Autodesk Inventor part; units mm, degrees
ref_plane "YZ Plane" through (0, 0, 0) normal (1, 0, 0) x (0, 1, 0)
ref_plane "XZ Plane" through (0, 0, 0) normal (0, 1, 0) x (-1, 0, 0)
ref_plane "XY Plane" through (0, 0, 0) normal (0, 0, 1) x (1, 0, 0)
sketch "Skizze1" plane through (0, 0, 0) normal (0, 1, 0) x (-1, 0, 0)
  line L0 (0, -10) -> (0, 10)
  line L1 (0, 10) -> (40, 10)
  line L2 (40, 10) -> (50, 0)
  line L3 (50, 0) -> (50, -7)
  line L4 (50, -7) -> (35, -7)
  line L5 (35, -7) -> (35, -10)
  line L6 (35, -10) -> (0, -10)
  line L7 (0, 0) -> (85.3703, 0) construction
  dimension "d0" = 10
  dimension "d1" = 10
  dimension "d2" = 3
  dimension "d3" = 20
  dimension "d4" = 40
  dimension "d5" = 15
extrude "Extrusion1" add sketch "Skizze1" along normal blind 60
sketch "Skizze2" plane through (-35, 0, -7) normal (0, 0, -1) x (-1, 0, 0)
  line L0 (15, 0) -> (15, 60)
  line L1 (15, 30) -> (5.3736, 30) construction
  line L2 (0, 60) -> (15, 60)
  point P0 (-35, 0)
  point P1 (8, 10)
  point P2 (8, 50)
  dimension "d8" = 7
  dimension "d9" = 7
  dimension "d10" = 40
  dimension "d11" = 10
hole "Bohrung1" at (-43, 10, -7) at (-43, 50, -7) direction (0, 0, 1) diameter 3.242 depth 12 tip angle 118
sketch "Skizze3" plane through (0, 0, -10) normal (0, 0, -1) x (-1, 0, 0)
  line L0 (0, 0) -> (0, 60)
  line L1 (0, 0) -> (35, 0)
  point P0 (20, 52)
  point P1 (20, 30)
  point P2 (20, 12)
  point P3 (0, 30)
  dimension "d19" = 20
  dimension "d20" = 12
  dimension "d21" = 40
hole "Bohrung2" at (-20, 12, -10) at (-20, 52, -10) direction (0, 0, 1) diameter 14 depth 20
hole "Bohrung3" at (-20, 30, -10) direction (0, 0, 1) diameter 13.835 depth 20
sketch "Skizze6" plane through (0, 0, 10) normal (1, 0, 0) x (0, 0, -1)
  line L0 (0, 60) -> (20, 60)
  point P0 (10, 0)
  point P1 (10, 54.0188)
  point P2 (10, 60)
hole "Bohrung4" at (0, 54.0188, 0) direction (-1, 0, 0) diameter 4.134 depth 10 tip angle 118
sketch "Skizze7" plane through (0, 0, 10) normal (1, 0, 0) x (0, 0, -1)
  line L0 (0, 0) -> (20, 0)
  point P0 (10, 0)
  point P1 (10, 10)
  point P2 (10, 0)
  point P3 (10, 0)
  dimension "d51" = 10
hole "Bohrung5" at (0, 10, 0) direction (-1, 0, 0) diameter 4.134 depth 10 tip angle 118
sketch "Skizze8" plane through (0, 0, 10) normal (1, 0, 0) x (0, 0, -1)
  line L0 (0, 0) -> (20, 0)
  point P0 (10, 0)
  point P1 (10, 30)
  point P2 (10, 0)
  point P3 (10, 0)
  point P4 (10, 0)
  dimension "d59" = 30
hole "Bohrung6" at (0, 30, 0) direction (-1, 0, 0) diameter 4.134 depth 10 tip angle 118
properties part number "spannbakce"
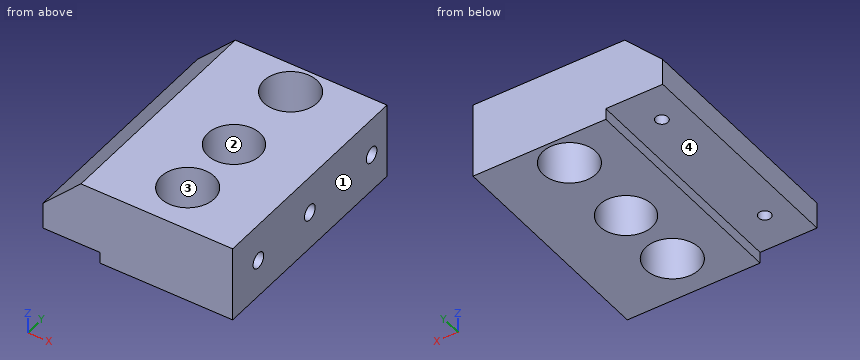
Can you work these out from the model? Positions are in its coordinate system, mm. Face numbers are marked on the shaded views. Coordinates: 2 decimals unless noted, no trailing zeros. Order: outer loops, then holes, each group sorted by start corner. A loop starts at its lowest first (then second) coordinate and runs counter-clockwise, first axis right, second up. Notation, with made-up numbers: (-4, -5.5) -> (0, -5.5) arc R17 cw to (0, 15.5) -> close; hole circle Ø3 at (-38.5, 48). An arc over 180 degrees is marked (long way). Use one line per item in the form item = value.
Q1. Will these pins go through, and if not, where does the flat tip stop? P1, Ø12.5, axis at x = -20, y = 30, coming from the -Z side; P2, Ø2, axis at x = -41.5, y = 30.5, coming from the -Z side; P3, Ø3, axis at y = 23, z = 4.5, coming from the -X side; P4, Ø3, axis at x = -43, y = 50, coming from the -Z side.
From the geometry:
P1 = through
P2 = -7
P3 = -47
P4 = 5.07
Q2. I need wall thicknesses on L1, parallel to Y at x = -20, z = -1.25; L2, parallel to Y at x = -2.75, z = 0; L3, parallel to Z at x = -5, y = 30. Which ranges of each line are inside material? Lowest first, please.
From the geometry:
L1 = 0 to 5, 19 to 23.08, 36.92 to 45, 59 to 60
L2 = 0 to 7.93, 12.07 to 27.93, 32.07 to 51.95, 56.09 to 60
L3 = -10 to -2.07, 2.07 to 10
Q3. Imagine slicing it at D-D, the plane z = 7.75. Give the number of separate pieces and of enclosed holes in the cut face, then the cut area to 3 significant figures.
From the geometry:
separate_pieces = 1
enclosed_holes = 3
area = 2,080 mm²
Q4. Imagine slicing it at A-A, the plane z = -5.5. List the corners of the cut face in (x, y) for me (1 decimal), then the cut area to 3 significant figures.
From the geometry:
outline = (-50, 0) -> (0, 0) -> (0, 60) -> (-50, 60) -> close; hole circle Ø3.2 at (-43, 10); hole circle Ø3.2 at (-43, 50); hole circle Ø14 at (-20, 12); hole circle Ø14 at (-20, 52); hole circle Ø13.8 at (-20, 30)
area = 2,530 mm²
Q5. Imagine slicing it at B-B, the plane x = -20. List the corners of the cut face in (y, z) for me, then the cut area to 3 significant figures.
From the geometry:
outline = (0, -10) -> (5, -10) -> (5, 10) -> (0, 10) -> close; (19, -10) -> (23.08, -10) -> (23.08, 10) -> (19, 10) -> close; (36.92, -10) -> (45, -10) -> (45, 10) -> (36.92, 10) -> close; (59, -10) -> (60, -10) -> (60, 10) -> (59, 10) -> close
area = 363 mm²
Q6. Imagine slicing it at C-C, the plane y = 22. List the corners of the cut face in (x, z) for me.
From the geometry:
outline = (-50, -7) -> (-35, -7) -> (-35, -10) -> (0, -10) -> (0, 10) -> (-40, 10) -> (-50, 0) -> close
Q7. We'd pull the mould along X, two halves only. Please class the marked faces 1, 2, 3 and 4: released by +X, released by -X, zero draft, split by the parting line, or undercut.
From the geometry:
face_1 = released by +X
face_2 = undercut
face_3 = undercut
face_4 = zero draft
